```python
from build123d import *
from build123d.topology import SkipClean

# Parameters (mm, degrees)
SKETCH1_R           = 4
SKETCH1_R_2         = 15
BOSS_EXTRUDE2_DEPTH = 5
SKETCH2_R           = 4
BOSS_EXTRUDE3_DEPTH = 30
BOSS_EXTRUDE4_START = 10
SKETCH4_R           = 30
SKETCH4_R_2         = 15
BOSS_EXTRUDE4_DEPTH = 10
BOSS_EXTRUDE6_START = -10
SKETCH7_R           = 3
BOSS_EXTRUDE6_DEPTH = 10
FILLET1_R           = 5
CUT_EXTRUDE2_START  = -10
SKETCH5_R           = 21
SKETCH5_R_2         = 15
CUT_EXTRUDE2_DEPTH  = 10
SKETCH8_R           = 18
CUT_EXTRUDE3_DEPTH  = 2
FILLET2_R           = 1
FILLET3_R           = 3


with BuildPart() as part:
    # Sketch1 → Boss-Extrude2 (new body)
    with BuildSketch(Plane.XY):
        with BuildLine():
            Line((-83.333333333, -10.859226218), (-83.333333333, -35.859226218))
            Line((-83.333333333, -35.859226218), (-83.333333333, -45.859226218))
            ThreePointArc((-83.333333333, -45.859226218), (-73.333333333, -55.859226218), (-63.333333333, -45.859226218))
            Line((-63.333333333, -45.859226218), (0, -45.859226218))
            Line((0, -45.859226218), (63.333333333, -45.859226218))
            ThreePointArc((63.333333333, -45.859226218), (73.333333333, -55.859226218), (83.333333333, -45.859226218))
            Line((83.333333333, -45.859226218), (83.333333333, -35.859226218))
            Line((83.333333333, -35.859226218), (83.333333333, -10.859226218))
            Line((83.333333333, -10.859226218), (32.135632545, -10.859226218))
            ThreePointArc((32.135632545, -10.859226218), (0, 33.920814748), (-32.135632545, -10.859226218))
            Line((-32.135632545, -10.859226218), (-83.333333333, -10.859226218))
        make_face()
        with Locations((-73.333333333, -45.859226218)):
            Circle(SKETCH1_R, mode=Mode.SUBTRACT)
        with Locations((73.333333333, -45.859226218)):
            Circle(SKETCH1_R, mode=Mode.SUBTRACT)
        Circle(SKETCH1_R_2, mode=Mode.SUBTRACT)
    extrude(amount=BOSS_EXTRUDE2_DEPTH)

    # Sketch2 → Boss-Extrude3 (add)
    # profile 1 of 2: a face of its own
    with BuildSketch(Plane.XY.offset(5)):
        with BuildLine():
            Line((83.333333333, -35.859226218), (-83.333333333, -35.859226218))
            Line((-83.333333333, -35.859226218), (-83.333333333, -45.859226218))
            ThreePointArc((-83.333333333, -45.859226218), (-73.333333333, -55.859226218), (-63.333333333, -45.859226218))
            Line((-63.333333333, -45.859226218), (63.333333333, -45.859226218))
            ThreePointArc((63.333333333, -45.859226218), (73.333333333, -55.859226218), (83.333333333, -45.859226218))
            Line((83.333333333, -45.859226218), (83.333333333, -35.859226218))
        make_face()
        with Locations((-73.333333333, -45.859226218)):
            Circle(SKETCH2_R, mode=Mode.SUBTRACT)
        with Locations((73.333333333, -45.859226218)):
            Circle(SKETCH2_R, mode=Mode.SUBTRACT)
    # profile 2 of 2: a face of its own
    with BuildSketch(Plane.XY.offset(5)):
        with BuildLine():
            Line((-83.333333333, -10.859226218), (-83.333333333, -15.859226218))
            Line((-83.333333333, -15.859226218), (-24.184674268, -15.859226218))
            ThreePointArc((-24.184674268, -15.859226218), (0, 28.920814748), (24.184674268, -15.859226218))
            Line((24.184674268, -15.859226218), (83.333333333, -15.859226218))
            Line((83.333333333, -15.859226218), (83.333333333, -10.859226218))
            Line((83.333333333, -10.859226218), (32.135632545, -10.859226218))
            ThreePointArc((32.135632545, -10.859226218), (0, 33.920814748), (-32.135632545, -10.859226218))
            Line((-32.135632545, -10.859226218), (-83.333333333, -10.859226218))
        make_face()
    extrude(amount=BOSS_EXTRUDE3_DEPTH)

    # Sketch4 → Boss-Extrude4 (add)
    with SkipClean():  # the faces are left unmerged after this step: merging them gives an invalid solid
        with BuildSketch(Plane(origin=(0, 0, 0), x_dir=(-1, 0, 0), z_dir=(0, 0, -1)).offset(BOSS_EXTRUDE4_START)):
            with Locations(Location((0, 0, 0), (0, 0, 180))):
                Circle(SKETCH4_R)
            Circle(SKETCH4_R_2, mode=Mode.SUBTRACT)
        extrude(amount=-BOSS_EXTRUDE4_DEPTH)

    # Sketch7 → Boss-Extrude6 (add)
    # profile 1 of 2: a face of its own
    with SkipClean():  # the faces are left unmerged after this step: merging them gives an invalid solid
        with BuildSketch(Plane.XY.offset(35).offset(BOSS_EXTRUDE6_START)):
            with BuildLine():
                Line((-46.135632545, -10.859226218), (-32.135632545, -10.859226218))
                ThreePointArc((-32.135632545, -10.859226218), (-33.685378506, -3.989604998), (-33.783237398, 3.051973795))
                ThreePointArc((-33.783237398, 3.051973795), (-48.189979587, 3.404653395), (-46.135632545, -10.859226218))
            make_face()
            with Locations((-41.135632545, -2.859226218)):
                Circle(SKETCH7_R, mode=Mode.SUBTRACT)
        # profile 2 of 2: a face of its own
        with BuildSketch(Plane.XY.offset(35).offset(BOSS_EXTRUDE6_START)):
            with BuildLine():
                Line((46.135632545, -10.859226218), (32.135632545, -10.859226218))
                ThreePointArc((32.135632545, -10.859226218), (33.685378506, -3.989604998), (33.783237398, 3.051973795))
                ThreePointArc((33.783237398, 3.051973795), (48.189979587, 3.404653395), (46.135632545, -10.859226218))
            make_face()
            with Locations((41.135632545, -2.859226218)):
                Circle(SKETCH7_R, mode=Mode.SUBTRACT)
        extrude(amount=BOSS_EXTRUDE6_DEPTH)

    # Fillet1
    fillet1_edges = [part.edges().sort_by_distance(p)[0] for p in [
        (-30, 0, -10),
    ]]
    fillet(fillet1_edges, radius=FILLET1_R)

    # Sketch5 → Cut-Extrude2 (cut)
    with BuildSketch(Plane.XY.offset(5).offset(CUT_EXTRUDE2_START)):
        Circle(SKETCH5_R)
        with Locations(Location((0, 0, 0), (0, 0, 180))):
            Circle(SKETCH5_R_2, mode=Mode.SUBTRACT)
    extrude(amount=CUT_EXTRUDE2_DEPTH, mode=Mode.SUBTRACT)

    # Sketch8 → Cut-Extrude3 (cut)
    with BuildSketch(Plane.XY.offset(-5)):
        Circle(SKETCH8_R)
    extrude(amount=-CUT_EXTRUDE3_DEPTH, mode=Mode.SUBTRACT)

    # Fillet2
    fillet2_edges = [part.edges().sort_by_distance(p)[0] for p in [
        (-73.333333333, -55.859226218, 0),
        (-83.333333333, -28.359226218, 0),
        (-57.734482939, -10.859226218, 0),
        (57.734482939, -10.859226218, 0),
        (83.333333333, -28.359226218, 0),
        (73.333333333, -55.859226218, 0),
        (0, -45.859226218, 0),
        (-83.333333333, -10.859226218, 17.5),
        (83.333333333, -10.859226218, 17.5),
    ]]
    fillet(fillet2_edges, radius=FILLET2_R)

    # Fillet3
    fillet3_edges = [part.edges().sort_by_distance(p)[0] for p in [
        (-24.184674268, -15.859226218, 20),
        (24.184674268, -15.859226218, 20),
    ]]
    fillet(fillet3_edges, radius=FILLET3_R)


solid = part.part
```
Can you work these out from the model? Positions are in its coordinate system, mm. A direction names the side the tool comes from. Coordinates: 2 decimals unless noted, no trailing zeros. Order: outer loops, then holes, each group sorted by start corner. A loop starts at its lowest first (then second) coordinate and runs counter-clockwise, first axis right, second up. Notation, with made-up numbers: (-18, 3.5) -> (16, 3.5) arc R5 cw to (16, 8.5) -> close; hole circle Ø3 at (-36, -15.75). An arc over 180 degrees is marked (long way). Write each question's results on one line, items separated by ' | '.
Item 1: I want a section at C-C, the plane z = 9.5. Write out the boundary of the cut face in (x, y), then the cut area to 3 significant figures.
Results are:
outline: (-83.33, -45.86) arc R10 ccw to (-63.33, -45.86) -> (63.33, -45.86) arc R10 ccw to (83.33, -45.86) -> (83.33, -35.86) -> (-83.33, -35.86) -> close; (-83.33, -15.86) -> (-29.22, -15.86) arc R3 ccw to (-26.47, -11.65) arc R28.92 cw (long way) to (26.47, -11.65) arc R3 ccw to (29.22, -15.86) -> (83.33, -15.86) -> (83.33, -11.86) arc R1 ccw to (82.33, -10.86) -> (32.14, -10.86) arc R33.92 ccw (long way) to (-32.14, -10.86) -> (-82.33, -10.86) arc R1 ccw to (-83.33, -11.86) -> close; hole circle Ø8 at (-73.33, -45.86); hole circle Ø8 at (73.33, -45.86) | area: 3,050 mm²
Item 2: I want a section at B-B, the plane z = 28.5. Write out the boundary of the cut face in (x, y).
Results are:
outline: (-83.33, -45.86) arc R10 ccw to (-63.33, -45.86) -> (63.33, -45.86) arc R10 ccw to (83.33, -45.86) -> (83.33, -35.86) -> (-83.33, -35.86) -> close; (-83.33, -15.86) -> (-29.22, -15.86) arc R3 ccw to (-26.47, -11.65) arc R28.92 cw (long way) to (26.47, -11.65) arc R3 ccw to (29.22, -15.86) -> (83.33, -15.86) -> (83.33, -11.86) arc R1 ccw to (82.33, -10.86) -> (46.14, -10.86) arc R9.43 ccw (long way) to (33.78, 3.05) arc R33.92 ccw to (-33.78, 3.05) arc R9.43 ccw (long way) to (-46.14, -10.86) -> (-82.33, -10.86) arc R1 ccw to (-83.33, -11.86) -> close; hole circle Ø8 at (-73.33, -45.86); hole circle Ø6 at (-41.14, -2.86); hole circle Ø6 at (41.14, -2.86); hole circle Ø8 at (73.33, -45.86)
Item 3: I want a section at A-A, the plane x = 0. Write out the boundary of the cut face in (y, z).
Results are:
outline: (-45.86, 1) arc R1 ccw to (-44.86, 0) -> (-30, 0) -> (-30, -5) arc R5 ccw to (-25, -10) -> (-15, -10) -> (-15, -7) -> (-18, -7) -> (-18, -5) -> (-21, -5) -> (-21, 5) -> (-35.86, 5) -> (-35.86, 35) -> (-45.86, 35) -> close; (15, -10) -> (25, -10) arc R5 ccw to (30, -5) -> (30, 0) -> (33.92, 0) -> (33.92, 35) -> (28.92, 35) -> (28.92, 5) -> (21, 5) -> (21, -5) -> (18, -5) -> (18, -7) -> (15, -7) -> close
Item 4: If we mould it in two halves opening along X, with no side actions, what happens to faces 1 (the face through (1, -35.859, 20)), 2 (the face through (-83.333, -36.2, 17.8)), 3 (the face through (20.03, 6.31, -0.07))? For each: +X half, -X half, draft (parallel to the pull), parting line (faces both ways), or undercut.
Results are:
face 1: draft | face 2: -X half | face 3: undercut
Item 5: Which directions (+Z, -Z, +X, -X, +Y, -Y) give clear straight access to the entire face, cutting with the end or side of a thin tool? Please do faces 4 (the face through (16.128, -25.296, -2.535)), 5 (the face through (-73.553, -55.857, 17.762)), 6 (the face through (-57, -15.859, 20)), 7 (the face through (11, 11, -10)), 8 (the face through (-2.343, 17.847, -5.986)).
Results are:
face 4: -Z | face 5: +Z, -Z, -Y | face 6: +Z, +X, -X | face 7: -Z, +X, -X, +Y, -Y | face 8: +Z
Item 6: I want a section at D-D, the plane y = -33. Write out the boundary of the cut face in (x, z).
Results are:
outline: (-83.33, 1) arc R1 ccw to (-82.33, 0) -> (82.33, 0) arc R1 ccw to (83.33, 1) -> (83.33, 5) -> (-83.33, 5) -> close
Item 7: If I drill on line 1 along Y through (x, z) = (58, 15.5); line 2 along Y through (x, z) = (1, 7.5); line 3 along X through (y, z) = (0, 23), over which ranges is the centre line in solid material (lowest first)?
Results are:
line 1: -45.86 to -35.86, -15.86 to -10.86 | line 2: -45.86 to -35.86, 28.9 to 33.91 | line 3: -33.92 to -28.92, 28.92 to 33.92
Item 8: I'm going to push flat-ended pins straight in: pin 1 Ø9.5 at (x, y) = (41.14, -2.86) entering from -Z; pin 2 Ø4 at (x, y) = (52.5, -24) entering from -Z; pin 3 Ø2 at (x, y) = (13.5, -22.5) entering from +Z. Where does each tip first touch, or does it pass through?
Results are:
pin 1: z = 25 | pin 2: z = 0 | pin 3: z = 5
